```python
from build123d import *

# Parameters (mm, degrees)
SKETCH1_R               = 18.25
SKETCH1_R_2             = 17.75
BOSS_EXTRUDE1_DEPTH     = 6.5
BOSS_EXTRUDE2_START     = -1.5
SKETCH2_R               = 18.25
BOSS_EXTRUDE2_DEPTH     = 1.5
BOSS_EXTRUDE3_START     = -0.5
SKETCH3_W               = 2.5
SKETCH3_H               = 6.738143646
BOSS_EXTRUDE3_DEPTH     = 1
SKETCH4_W               = 8
SKETCH4_H               = 2
BOSS_EXTRUDE4_DEPTH     = 8
FILLET1_R               = 2
CUT_EXTRUDE1_DEPTH      = 34.430553991
CUT_EXTRUDE1_DEPTH_BACK = 34.430553991
SKETCH5_R               = 1.5
FILLET2_R               = 2


with BuildPart() as part:
    # Sketch1 → Boss-Extrude1 (new body)
    with BuildSketch(Plane(origin=(0, 0, 0), x_dir=(1, 0, 0), z_dir=(0, 1, 0))):
        with Locations(Location((0, 0, 0), (0, 0, 90))):
            Circle(SKETCH1_R)
        with Locations(Location((0, 0, 0), (0, 0, 90))):
            Circle(SKETCH1_R_2, mode=Mode.SUBTRACT)
    extrude(amount=BOSS_EXTRUDE1_DEPTH)

    # Sketch2 → Boss-Extrude2 (add)
    with BuildSketch(Plane(origin=(0, 6.5, 0), x_dir=(1, 0, 0), z_dir=(0, 1, 0)).offset(BOSS_EXTRUDE2_START)):
        with Locations(Location((0, 0, 0), (0, 0, 90))):
            Circle(SKETCH2_R)
    extrude(amount=BOSS_EXTRUDE2_DEPTH)

    # Sketch3 → Boss-Extrude3 (add)
    with BuildSketch(Plane(origin=(0, 5, 0), x_dir=(-1, 0, 0), z_dir=(0, -1, 0)).offset(BOSS_EXTRUDE3_START)):
        Polygon((18.622786456, -12.318351976), (12.787382884, -8.949280153), (14.037382884, -6.784216644), (19.872786456, -10.153288467), align=None)
        with Locations((0, 18.97946309)):
            Rectangle(SKETCH3_W, SKETCH3_H)
        Polygon((-20.086011489, -10.030182937), (-14.250607917, -6.661111114), (-13.000607917, -8.826174624), (-18.836011489, -12.195246447), align=None)
    extrude(amount=-BOSS_EXTRUDE3_DEPTH)

    # Sketch4 → Boss-Extrude4 (add)
    with BuildSketch(Plane(origin=(0, 5, 0), x_dir=(-1, 0, 0), z_dir=(0, -1, 0))):
        Rectangle(SKETCH4_W, SKETCH4_H)
    extrude(amount=-BOSS_EXTRUDE4_DEPTH)

    # Fillet1
    fillet1_edges = [part.edges().sort_by_distance(p)[0] for p in [
        (-4, 6.5, 0),
        (0, 6.5, 1),
        (4, 6.5, 0),
        (0, 6.5, -1),
    ]]
    fillet(fillet1_edges, radius=FILLET1_R)

    # Sketch5 → Cut-Extrude1 (cut, two sides: drawn at the far end of the back side and taken through both)
    with BuildSketch(Plane.XY.offset(1).offset(-CUT_EXTRUDE1_DEPTH_BACK)):
        with Locations(Location((0, 9.597763348, 0), (0, 0, 312.958942011))):
            Circle(SKETCH5_R)
    extrude(amount=CUT_EXTRUDE1_DEPTH + CUT_EXTRUDE1_DEPTH_BACK, mode=Mode.SUBTRACT)

    # Fillet2
    fillet2_edges = [part.edges().sort_by_distance(p)[0] for p in [
        (-4, 13, 0),
        (4, 13, 0),
    ]]
    fillet(fillet2_edges, radius=FILLET2_R)


solid = part.part
```
CAD build for the part. Positions are in the model's coordinates, mm. A direction names the side the tool comes from. Round coordinates to 2 decimals unless told otherwise and drop trailing zeros. Write each loop counter-clockwise with the first axis right and the second up, starting at its lowest first coordinate (ties: lowest second). Pieces come first, ordered by that corner, then holes. Notation, with made-up numbers: (-26, 6) -> (-2, 6) arc R26 ccw to (-2, 41) -> close; hole circle Ø8 at (60.5, 46.25). An arc over 180 degrees is marked (long way). Answer in a Markdown table with one row per item. Add a question column.
Item 1: Saw through at D-D, the plane y = 3.75. Write the cut outline in (x, z).
Item 2: Saw through at A-A, the plane x = 0. Write the cut outline in (y, z).
Item 3: Saw through at B-B, the plane y = 9.5. Write the cut outline in (x, z).
Item 4: Which spindle directions (+Z, -Z, +X, -X, +Y, -Y) get a long thin tool onto all of the face, cutting with end or side? Do faces 4 (the face through (4, 10, 0)), 5 (the face through (-18, 5.5, 10)), 6 (the face through (15.747, 2.465, -8.191)). Say none if no direction does.
Item 5: Drill centre lines: line 1 (Y direction, x = 0, z = -0.05); line 2 (X direction, y = 3.5, z = 0); line 3 (Y direction, x = -5, z = -12). Where is each one in solid material? Low to high. Write a range as from..to.
Item 6: Mould opens along Z. For faces 1 (the face through (0, 12, 1)), 2 (the face through (-18.08, 5.99, 9.12)), 3 (the face through (18, 5.5, 10)) say: pulls with the +Z half, pulls with the -Z half, needs draft (parallel to the pull), parting line crosses it, or undercut.
Item 7: Drop flat-ended pins along their axis: pin 1 Ø3 at (x, z) = (0, -20) entering from -Y; pin 2 Ø5 at (x, y) = (1.5, 11) entering from -Z; pin 3 Ø1.3 at (x, y) = (-0.5, 11.5) entering from +Z. Give the stop position or say it passes through.
Item 8: Saw through at C-C, the plane z = 0. Write the cut outline in (x, y), then the cut area to 3 significant figures.
Findings below:
| question | item | result |
|---|---|---|
| 1 | outline | circle Ø36.5 at (0, 0); hole circle Ø35.5 at (0, 0) |
| 2 | outline | (0, -18.25) -> (5.5, -18.25) -> (5.5, -22.35) -> (6.5, -22.35) -> (6.5, -3) arc R2 cw to (8.1, -1.04) -> (8.1, 1.04) arc R2 cw to (6.5, 3) -> (6.5, 18.25) -> (0, 18.25) -> (0, 17.75) -> (5, 17.75) -> (5, -17.75) -> (0, -17.75) -> close; (11.1, -1) -> (13, -1) -> (13, 1) -> (11.1, 1) -> close |
| 3 | outline | (-4, -1) -> (-1.5, -1) -> (-1.5, 1) -> (-4, 1) -> close; (1.5, -1) -> (4, -1) -> (4, 1) -> (1.5, 1) -> close |
| 4 | face 4 | +Z, -Z, +X, +Y |
| 4 | face 5 | +Z, -X, -Y |
| 4 | face 6 | -Y |
| 5 | line 1 | y = 5..8.1, 11.1..13 |
| 5 | line 2 | x = -18.25..-17.75, 17.75..18.25 |
| 5 | line 3 | y = 5..6.5 |
| 6 | face 1 | pulls with the +Z half |
| 6 | face 2 | undercut |
| 6 | face 3 | needs draft |
| 7 | pin 1 | stops at y = 5.5 |
| 7 | pin 2 | stops at z = -1 |
| 7 | pin 3 | stops at z = 1 |
| 8 | outline | (-18.25, 0) -> (-17.75, 0) -> (-17.75, 5) -> (17.75, 5) -> (17.75, 0) -> (18.25, 0) -> (18.25, 6.5) -> (6, 6.5) arc R2 cw to (4, 8.5) -> (4, 11) arc R2 ccw to (2, 13) -> (-2, 13) arc R2 ccw to (-4, 11) -> (-4, 8.5) arc R2 cw to (-6, 6.5) -> (-18.25, 6.5) -> close; hole circle Ø3 at (0, 9.6) |
| 8 | area | 105 mm^2 |
